from build123d import *

# Parameters (mm, degrees)
PAD_DEPTH       = 27
POCKET_DEPTH    = 21
POCKET005_DEPTH = 5
SKETCH015_W     = 6
SKETCH015_H     = 11
SKETCH015_W_2   = 8
PAD006_DEPTH    = 15.5
SKETCH012_W     = 3
SKETCH012_H     = 3
SKETCH012_W_2   = 10
SKETCH012_W_3   = 11
PAD007_DEPTH    = 24
SKETCH016_R     = 1.7
HOLE_DEPTH      = 11.5
HOLE_TIPS_R     = 1.7
SKETCH017_R     = 1.7
HOLE001_DEPTH   = 20
HOLE001_TIPS_R  = 1.7
SKETCH018_W     = 36
SKETCH018_H     = 36
PAD008_DEPTH    = 2
SKETCH025_R     = 1.7
POCKET010_DEPTH = 1
SKETCH028_W     = 88
SKETCH028_H     = 2
POCKET011_DEPTH = 115.001
CHAMFER_SIZE    = 0.5


with BuildPart() as part:
    # Sketch → Pad (new body)
    with BuildSketch(Plane.XY):
        Polygon((-5, -7), (70, -7), (78, -17), (110, -17), (110, 71), (-5, 71), align=None)
    extrude(amount=PAD_DEPTH)

    # Sketch001 (on Face8 of Pad) → Pocket (cut)
    with BuildSketch(Plane.XY.offset(27)):
        Polygon((0, 66), (0, -2), (71, -2), (79, -12), (105, -12), (105, 66), align=None)
    extrude(amount=-POCKET_DEPTH, mode=Mode.SUBTRACT)

    # Sketch014 → Pocket005 (cut)
    with BuildSketch(Plane.YZ.offset(110)):
        with BuildLine():
            ThreePointArc((56.25908, 12.405), (53, 24.475), (49.74092, 12.405))
            Line((49.74092, 12.405), (56.25908, 12.405))
        make_face()
        with BuildLine():
            ThreePointArc((4.746425, 15.2), (3, 21.3), (1.253575, 15.2))
            Line((4.746425, 15.2), (1.253575, 15.2))
        make_face()
        with BuildLine():
            ThreePointArc((22.65, 15.069556), (28, 11.9), (33.35, 15.069556))
            Line((33.35, 20.930444), (33.35, 15.069556))
            ThreePointArc((33.35, 20.930444), (28, 24.1), (22.65, 20.930444))
            Line((22.65, 20.930444), (22.65, 15.069556))
        make_face()
    extrude(amount=-POCKET005_DEPTH, mode=Mode.SUBTRACT)

    # Sketch015 → Pad006 (join)
    with BuildSketch(Plane.XY.offset(3)):
        with Locations((3, 61.5)):
            Rectangle(SKETCH015_W, SKETCH015_H)
        with Locations((78, 61.5)):
            Rectangle(SKETCH015_W_2, SKETCH015_H)
    extrude(amount=PAD006_DEPTH)

    # Sketch012 → Pad007 (join)
    with BuildSketch(Plane.XY.offset(3)):
        with Locations((1.5, 64.5)):
            Rectangle(SKETCH012_W, SKETCH012_H)
        with Locations((103.5, 64.5)):
            Rectangle(SKETCH012_W, SKETCH012_H)
        with Locations((103.5, -10.5)):
            Rectangle(SKETCH012_W, SKETCH012_H)
        with Locations((1.5, -0.5)):
            Rectangle(SKETCH012_W, SKETCH012_H)
        with Locations((66, 64.5)):
            Rectangle(SKETCH012_W_2, SKETCH012_H)
        with Locations((32, -0.5)):
            Rectangle(SKETCH012_W_2, SKETCH012_H)
        with Locations((66, -0.5)):
            Rectangle(SKETCH012_W_2, SKETCH012_H)
        with Locations((32.5, 64.5)):
            Rectangle(SKETCH012_W_3, SKETCH012_H)
    extrude(amount=PAD007_DEPTH)

    # Sketch016 → Hole (cut)
    with BuildSketch(Plane.XY.offset(18.5)):
        with Locations((3.25, 59)):
            Circle(SKETCH016_R)
        with Locations((77, 59)):
            Circle(SKETCH016_R)
    extrude(amount=-HOLE_DEPTH, mode=Mode.SUBTRACT)

    # Hole tips → Hole tip 1 section 0
    with BuildSketch(Plane.XY.offset(7), mode=Mode.PRIVATE) as hole_tip_1_s0:
        with Locations((3.25, 59)):
            Circle(HOLE_TIPS_R)
    loft([hole_tip_1_s0.sketch, Vertex(3.25, 59, 5.978537)], mode=Mode.SUBTRACT)

    # Hole tips → Hole tip 2 section 0
    with BuildSketch(Plane.XY.offset(7), mode=Mode.PRIVATE) as hole_tip_2_s0:
        with Locations((77, 59)):
            Circle(HOLE_TIPS_R)
    loft([hole_tip_2_s0.sketch, Vertex(77, 59, 5.978537)], mode=Mode.SUBTRACT)

    # Sketch017 (on Face2 of Hole) → Hole001 (cut)
    with BuildSketch(Plane.XY.offset(27)):
        with Locations((-1, 67)):
            Circle(SKETCH017_R)
        with Locations((106, 67)):
            Circle(SKETCH017_R)
        with Locations((106, -13)):
            Circle(SKETCH017_R)
        with Locations((-1, -3)):
            Circle(SKETCH017_R)
        with Locations((66, 67)):
            Circle(SKETCH017_R)
        with Locations((66, -3)):
            Circle(SKETCH017_R)
        with Locations((32, -3)):
            Circle(SKETCH017_R)
        with Locations((32, 67)):
            Circle(SKETCH017_R)
    extrude(amount=-HOLE001_DEPTH, mode=Mode.SUBTRACT)

    # Hole001 tips → Hole001 tip 1 section 0
    with BuildSketch(Plane.XY.offset(7), mode=Mode.PRIVATE) as hole001_tip_1_s0:
        with Locations((-1, 67)):
            Circle(HOLE001_TIPS_R)
    loft([hole001_tip_1_s0.sketch, Vertex(-1, 67, 5.978537)], mode=Mode.SUBTRACT)

    # Hole001 tips → Hole001 tip 2 section 0
    with BuildSketch(Plane.XY.offset(7), mode=Mode.PRIVATE) as hole001_tip_2_s0:
        with Locations((106, 67)):
            Circle(HOLE001_TIPS_R)
    loft([hole001_tip_2_s0.sketch, Vertex(106, 67, 5.978537)], mode=Mode.SUBTRACT)

    # Hole001 tips → Hole001 tip 3 section 0
    with BuildSketch(Plane.XY.offset(7), mode=Mode.PRIVATE) as hole001_tip_3_s0:
        with Locations((106, -13)):
            Circle(HOLE001_TIPS_R)
    loft([hole001_tip_3_s0.sketch, Vertex(106, -13, 5.978537)], mode=Mode.SUBTRACT)

    # Hole001 tips → Hole001 tip 4 section 0
    with BuildSketch(Plane.XY.offset(7), mode=Mode.PRIVATE) as hole001_tip_4_s0:
        with Locations((-1, -3)):
            Circle(HOLE001_TIPS_R)
    loft([hole001_tip_4_s0.sketch, Vertex(-1, -3, 5.978537)], mode=Mode.SUBTRACT)

    # Hole001 tips → Hole001 tip 5 section 0
    with BuildSketch(Plane.XY.offset(7), mode=Mode.PRIVATE) as hole001_tip_5_s0:
        with Locations((66, 67)):
            Circle(HOLE001_TIPS_R)
    loft([hole001_tip_5_s0.sketch, Vertex(66, 67, 5.978537)], mode=Mode.SUBTRACT)

    # Hole001 tips → Hole001 tip 6 section 0
    with BuildSketch(Plane.XY.offset(7), mode=Mode.PRIVATE) as hole001_tip_6_s0:
        with Locations((66, -3)):
            Circle(HOLE001_TIPS_R)
    loft([hole001_tip_6_s0.sketch, Vertex(66, -3, 5.978537)], mode=Mode.SUBTRACT)

    # Hole001 tips → Hole001 tip 7 section 0
    with BuildSketch(Plane.XY.offset(7), mode=Mode.PRIVATE) as hole001_tip_7_s0:
        with Locations((32, -3)):
            Circle(HOLE001_TIPS_R)
    loft([hole001_tip_7_s0.sketch, Vertex(32, -3, 5.978537)], mode=Mode.SUBTRACT)

    # Hole001 tips → Hole001 tip 8 section 0
    with BuildSketch(Plane.XY.offset(7), mode=Mode.PRIVATE) as hole001_tip_8_s0:
        with Locations((32, 67)):
            Circle(HOLE001_TIPS_R)
    loft([hole001_tip_8_s0.sketch, Vertex(32, 67, 5.978537)], mode=Mode.SUBTRACT)

    # Sketch018 → Pad008 (join)
    with BuildSketch(Plane.XY.offset(6)):
        with Locations((40, 23)):
            Rectangle(SKETCH018_W, SKETCH018_H)
    extrude(amount=PAD008_DEPTH)

    # Sketch025 → Pocket010 (cut)
    with BuildSketch(Plane.XY.offset(27)):
        with BuildLine():
            ThreePointArc((109, 67), (108.12132, 69.12132), (106, 70))
            Line((-1, 70), (106, 70))
            ThreePointArc((-1, 70), (-3.12132, 69.12132), (-4, 67))
            Line((-4, -3), (-4, 67))
            ThreePointArc((-4, -3), (-3.12132, -5.12132), (-1, -6))
            Line((-1, -6), (70.5, -6))
            Line((70.5, -6), (78.5, -16))
            Line((78.5, -16), (106, -16))
            ThreePointArc((106, -16), (108.12132, -15.12132), (109, -13))
            Line((109, 67), (109, -13))
        make_face()
        with Locations((32, 67)):
            Circle(SKETCH025_R, mode=Mode.SUBTRACT)
        with Locations((32, -3)):
            Circle(SKETCH025_R, mode=Mode.SUBTRACT)
        with BuildLine():
            Line((107, -10.171573), (107, 64.171573))
            ThreePointArc((103.171573, 68), (103.87868, 64.87868), (107, 64.171573))
            Line((68.828427, 68), (103.171573, 68))
            ThreePointArc((63.171573, 68), (66, 64), (68.828427, 68))
            Line((34.828427, 68), (63.171573, 68))
            ThreePointArc((29.171573, 68), (32, 64), (34.828427, 68))
            Line((1.828427, 68), (29.171573, 68))
            ThreePointArc((-2, 64.171573), (1.12132, 64.87868), (1.828427, 68))
            Line((-2, 64.171573), (-2, -0.171573))
            ThreePointArc((1.828427, -4), (1.12132, -0.87868), (-2, -0.171573))
            Line((29.171573, -4), (1.828427, -4))
            ThreePointArc((34.828427, -4), (32, 0), (29.171573, -4))
            Line((63.171573, -4), (34.828427, -4))
            ThreePointArc((68.828427, -4), (66, 0), (63.171573, -4))
            Line((71, -4), (68.828427, -4))
            Line((79, -14), (71, -4))
            Line((103.171573, -14), (79, -14))
            ThreePointArc((107, -10.171573), (103.87868, -10.87868), (103.171573, -14))
        make_face(mode=Mode.SUBTRACT)
    extrude(amount=-POCKET010_DEPTH, mode=Mode.SUBTRACT)

    # Sketch028 (on Face92 of Pocket010) → Pocket011 (cut, through all)
    with BuildSketch(Plane.YZ.offset(110)):
        with Locations((27, 1)):
            Rectangle(SKETCH028_W, SKETCH028_H)
    extrude(amount=-POCKET011_DEPTH, mode=Mode.SUBTRACT)

    # Chamfer
    chamfer_edges = [part.edges().sort_by_distance(p)[0] for p in [
        (110, -17, 14.5),
        (110, 27, 2),
        (52.5, 71, 2),
        (110, 71, 14.5),
        (32.5, -7, 2),
        (94, -17, 2),
        (74, -12, 2),
        (-5, -7, 14.5),
        (-5, 32, 2),
        (-5, 71, 14.5),
    ]]
    chamfer(chamfer_edges, length=CHAMFER_SIZE)


with BuildPart() as part_1:
    # Body placement: moved
    add(part.part.moved(Location((0, 0, -2.5))))


solid = part_1.part
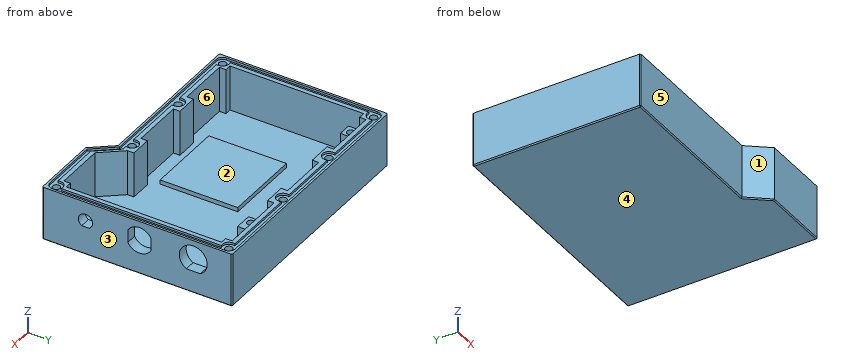
CAD build for the part. Positions are in the model's coordinates, mm. Face numbers are marked on the shaded views. A direction names the side the tool comes from. Coordinates: 2 decimals unless noted, no trailing zeros. Order: outer loops, then holes, each group sorted by start corner. A loop starts at its lowest first (then second) coordinate and runs counter-clockwise, first axis right, second up. Notation, with made-up numbers: (82, -9.75) -> (126, -9.75) arc R20 ccw to (126, 25.25) -> close; hole circle Ø10 at (61.5, -21). An arc over 180 degrees is marked (long way). Answer in a Markdown table with one row per item.
1) Band-saw the part on C-C (x = 51). List the corners of the cut face in (y, z), and give its area (3 significant figures).
Check values:
| item | result |
|---|---|
| outline | (-7, 0) -> (-6.5, -0.5) -> (70.5, -0.5) -> (71, 0) -> (71, 24.5) -> (70, 24.5) -> (70, 23.5) -> (68, 23.5) -> (68, 24.5) -> (66, 24.5) -> (66, 3.5) -> (41, 3.5) -> (41, 5.5) -> (5, 5.5) -> (5, 3.5) -> (-2, 3.5) -> (-2, 24.5) -> (-4, 24.5) -> (-4, 23.5) -> (-6, 23.5) -> (-6, 24.5) -> (-7, 24.5) -> close |
| area | 590 mm2 |
2) Band-saw the part on B-B (z = 1.5). List the corners of the cut face in (x, y).
Check values:
| item | result |
|---|---|
| outline | (-5, -6.5) -> (-4.5, -7) -> (70, -7) -> (78, -17) -> (109.5, -17) -> (110, -16.5) -> (110, 70.5) -> (109.5, 71) -> (-4.5, 71) -> (-5, 70.5) -> close |
3) Band-saw the part on A-A (y = 53). List the corners of the cut face in (x, z) (3 decimals), and give its area (3 significant figures).
Check values:
| item | result |
|---|---|
| outline | (-5, 0) -> (-4.5, -0.5) -> (109.5, -0.5) -> (110, 0) -> (110, 9.905) -> (105, 9.905) -> (105, 3.5) -> (0, 3.5) -> (0, 24.5) -> (-2, 24.5) -> (-2, 23.5) -> (-4, 23.5) -> (-4, 24.5) -> (-5, 24.5) -> close; (105, 21.975) -> (110, 21.975) -> (110, 24.5) -> (109, 24.5) -> (109, 23.5) -> (107, 23.5) -> (107, 24.5) -> (105, 24.5) -> close |
| area | 605 mm2 |
4) Mould opens along Y. For the marked faces 1, 2 and 3 say: pulls with the +Y half, pulls with the -Y half, needs draft (parallel to the pull), parting line crosses it, or undercut.
Check values:
| item | result |
|---|---|
| face 1 | pulls with the -Y half |
| face 2 | undercut |
| face 3 | needs draft |
5) Drill centre lines: line 1 (X direction, y = 67, z = 18); line 2 (Y direction, x = 66, z = 23.7); line 3 (X direction, y = 67, z = 24.1). Where is each one in solid material? Low to high.
Check values:
| item | result |
|---|---|
| line 1 | -5 to -2.7, 0.7 to 30.3, 33.7 to 64.3, 67.7 to 104.3, 107.7 to 110 |
| line 2 | -7 to -6, 0 to 1, 63 to 64, 70 to 71 |
| line 3 | -5 to -4, 2 to 29, 35 to 63, 69 to 103, 109 to 110 |
6) Flat gauge pins, fed straight in: P1, Ø10.5, axis at x = 18, z = 9, coming from the -Y side; P2, Ø4, axis at x = 17.5, y = 54.5, coming from the +Z side; P3, Ø2, axis at x = 44, y = 6, coming from the +Z side. Where does each tip first touch, or does it go through?
Check values:
| item | result |
|---|---|
| P1 | y = -7 |
| P2 | z = 3.5 |
| P3 | z = 5.5 |
7) Which spindle directions (+Z, -Z, +X, -X, +Y, -Y) get a long thin tool onto all of the face, cutting with end or side? Do the marked faces 4, 5 and 6. Say none if no direction does.
Check values:
| item | result |
|---|---|
| face 4 | -Z, +X, -X, +Y, -Y |
| face 5 | +Z, -Z, -X, -Y |
| face 6 | +Z |
